Input: part model. Units: mm. Frame: model coordinates. Face numbers are marked on the shaded views. A direction names the side the tool comes from. Round coordinates to 2 decimals unless told otherwise and drop trailing zeros. Loops run counter-clockwise (first coordinate to the right, second up) from the corner with the lowest first, then second, coordinate; pieces in that order, holes last.
1) Ray query, line 1 along X through (y, z) = (-8, 4); line 2 along Y through (x, z) = (-4.75, 4.5); line 3 along Y through (x, z) = (-4, 5). Return the intervals inside material, ascending.
2) Section C-C, the plane x = 2. Return loops of the section in (y, z) (1 decimal).
3) Section A-A, the plane y = 12.5. Return loops of the section in (x, z), and give its area (3 significant figures).
4) Draft query along X for the marked faces 4, 5, 6 and 7. Return one class per face: pulls with the +X half, pulls with the -X half, needs draft (parallel to the pull), parting line crosses it, or undercut.
5) Access query for the marked faces 1, 2 and 3. Directions: +Z, -Z, +X, -X, +Y, -Y. A direction counts if a zero-diameter tool reaches every point of the face in a straight line with its end or side. Return the directions, or none.
6) Section B-B, the plane z = 6. Return loops of the section in (x, y) (3 decimals).
7) Section D-D, the plane y = -20.5. Return loops of the section in (x, z).
8) First-contact query: pin 1 (1.3 mm diameter, centred on x = 3, y = -27, fed in from -Z); pin 2 (6 mm diameter, centred on x = 1.85, y = -27.42, fed in from +Z); pin 3 (5 mm diameter, centred on x = 3, z = 2, fed in from +Y); pin 4 (3 mm diameter, centred on y = 28.5, z = 5.5, fed in from -X). Flat tips, straight axial feed; report the tip coordinate or a pass-through.
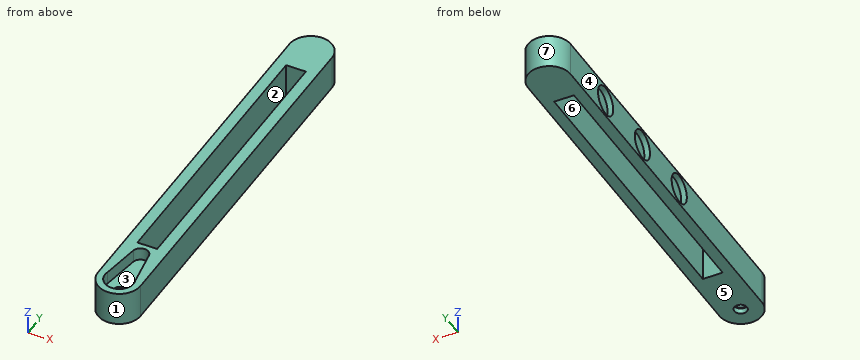
from build123d import *

# Parameters (mm, degrees)
BOSS_EXTRUDE1_DEPTH = 12
SKETCH5_W           = 7
SKETCH5_H           = 112.5
CUT_EXTRUDE3_DEPTH  = 12
SKETCH6_R           = 5.15
CUT_EXTRUDE4_DEPTH  = 2
SKETCH7_W           = 9.454853554
SKETCH7_H           = 12.627623204
BOSS_EXTRUDE2_DEPTH = 12
SKETCH8_R           = 1.8
CUT_EXTRUDE5_DEPTH  = 4.5
SKETCH9_R           = 1.8
CUT_EXTRUDE6_DEPTH  = 13.5
SKETCH10_R          = 2.25
CUT_EXTRUDE7_DEPTH  = 2


with BuildPart() as part:
    # Sketch1 → Boss-Extrude1 (new body)
    with BuildSketch(Plane.XY):
        with BuildLine():
            Line((-5.64516129, 102.580645161), (-5.64516129, -27.419354839))
            ThreePointArc((-5.64516129, -27.419354839), (1.85483871, -34.919354839), (9.35483871, -27.419354839))
            Line((9.35483871, -27.419354839), (9.35483871, 102.580645161))
            ThreePointArc((9.35483871, 102.580645161), (1.85483871, 110.080645161), (-5.64516129, 102.580645161))
        make_face()
    extrude(amount=BOSS_EXTRUDE1_DEPTH)

    # Sketch5 → Cut-Extrude3 (cut)
    with BuildSketch(Plane.XY.offset(12)):
        with Locations((1.85483871, 36.330645161)):
            Rectangle(SKETCH5_W, SKETCH5_H)
    extrude(amount=-CUT_EXTRUDE3_DEPTH, mode=Mode.SUBTRACT)

    # Sketch6 → Cut-Extrude4 (cut)
    with BuildSketch(Plane.ZY.offset(5.64516129)):
        with Locations((6, 78.768969581)):
            Circle(SKETCH6_R)
        with Locations((6, 53.768969581)):
            Circle(SKETCH6_R)
        with Locations((6, 28.768969581)):
            Circle(SKETCH6_R)
    extrude(amount=-CUT_EXTRUDE4_DEPTH, mode=Mode.SUBTRACT)

    # Sketch7 → Boss-Extrude2 (add)
    with BuildSketch(Plane.XY.offset(12)):
        with Locations((2.35113594, -14.728820961)):
            Rectangle(SKETCH7_W, SKETCH7_H)
    extrude(amount=-BOSS_EXTRUDE2_DEPTH)

    # Sketch8 → Cut-Extrude5 (cut)
    with BuildSketch(Plane.XY.offset(12)):
        with BuildLine():
            Line((6.693784724, -25.961716652), (4.61141034, -12.592472516))
            ThreePointArc((4.61141034, -12.592472516), (1.845305929, -10.267914611), (-0.920798482, -12.592472516))
            Line((-0.920798482, -12.592472516), (-2.997287431, -26.006209578))
            ThreePointArc((-2.997287431, -26.006209578), (1.878040737, -32.473023732), (6.693784724, -25.961716652))
        make_face()
        with Locations((1.85483871, -27.419354839)):
            Circle(SKETCH8_R, mode=Mode.SUBTRACT)
    extrude(amount=-CUT_EXTRUDE5_DEPTH, mode=Mode.SUBTRACT)

    # Sketch9 → Cut-Extrude6 (cut)
    with BuildSketch(Plane.XY.offset(12)):
        with Locations((1.85483871, -27.419354839)):
            Circle(SKETCH9_R)
    extrude(amount=-CUT_EXTRUDE6_DEPTH, mode=Mode.SUBTRACT)

    # Sketch10 → Cut-Extrude7 (cut)
    with BuildSketch(Plane(origin=(0, 0, 0), x_dir=(-1, 0, 0), z_dir=(0, 0, -1))):
        with Locations((-1.85483871, -27.419354839)):
            Circle(SKETCH10_R)
    extrude(amount=-CUT_EXTRUDE7_DEPTH, mode=Mode.SUBTRACT)


solid = part.part
Final values:
1. line 1: x = -5.65 to -1.65, 5.35 to 9.35
1. line 2: y = -30.97 to 23.84, 33.7 to 48.84, 58.7 to 73.84, 83.7 to 106.13
1. line 3: y = -32.11 to 23.72, 33.82 to 48.72, 58.82 to 73.72, 83.82 to 107.27
2. outline: (-34.9, 0) - (-29.7, 0) - (-29.7, 2) - (-29.2, 2) - (-29.2, 7.5) - (-32.5, 7.5) - (-32.5, 12) - (-34.9, 12) - close; (-25.6, 2) - (-25.2, 2) - (-25.2, 0) - (-8.4, 0) - (-8.4, 12) - (-10.3, 12) - (-10.3, 7.5) - (-25.6, 7.5) - close; (92.6, 0) - (110.1, 0) - (110.1, 12) - (92.6, 12) - close
3. outline: (-5.65, 0) - (-1.65, 0) - (-1.65, 12) - (-5.65, 12) - close; (5.35, 0) - (9.35, 0) - (9.35, 12) - (5.35, 12) - close
3. area: 96.0 mm2
4. face 4: pulls with the -X half
4. face 5: needs draft
4. face 6: undercut
4. face 7: parting line crosses it
5. face 1: +Z, -Z, -Y
5. face 2: +Z, -Z
5. face 3: +Z
6. outline: (-5.645, -27.419) arc R7.5 ccw to (9.355, -27.419) - (9.355, 102.581) arc R7.5 ccw to (-5.645, 102.581) - (-5.645, 83.919) - (-3.645, 83.919) - (-3.645, 73.619) - (-5.645, 73.619) - (-5.645, 58.919) - (-3.645, 58.919) - (-3.645, 48.619) - (-5.645, 48.619) - (-5.645, 33.919) - (-3.645, 33.919) - (-3.645, 23.619) - (-5.645, 23.619) - close; hole (-1.645, -8.415) - (5.355, -8.415) - (5.355, 92.581) - (-1.645, 92.581) - close; hole circle Ø3.6 at (1.855, -27.419)
7. outline: (-5.65, 0) - (9.35, 0) - (9.35, 12) - (5.84, 12) - (5.84, 7.5) - (-2.14, 7.5) - (-2.14, 12) - (-5.65, 12) - close
8. pin 1: stops at z = 2
8. pin 2: stops at z = 7.5
8. pin 3: stops at y = 110.08
8. pin 4: stops at x = -3.65
